```python
from build123d import *

# Parameters (mm, degrees)
SKETCH1_W           = 10
SKETCH1_H           = 7
BOSS_EXTRUDE1_DEPTH = 2
SKETCH2_W           = 7
SKETCH2_H           = 10
BOSS_EXTRUDE2_DEPTH = 2
SKETCH3_R           = 1.05
CUT_EXTRUDE1_DEPTH  = 14.275918047
SKETCH4_R           = 1.05
CUT_EXTRUDE2_DEPTH  = 14.275918047
FILLET1_R           = 1


with BuildPart() as part:
    # Sketch1 → Boss-Extrude1 (new body)
    with BuildSketch(Plane(origin=(0, 0, 0), x_dir=(1, 0, 0), z_dir=(0, 1, 0))):
        with Locations((-5, 0)):
            Rectangle(SKETCH1_W, SKETCH1_H)
    extrude(amount=BOSS_EXTRUDE1_DEPTH)

    # Sketch2 → Boss-Extrude2 (add)
    with BuildSketch(Plane(origin=(0, 0, 0), x_dir=(0, 0, -1), z_dir=(1, 0, 0))):
        with Locations((0, 5)):
            Rectangle(SKETCH2_W, SKETCH2_H)
    extrude(amount=-BOSS_EXTRUDE2_DEPTH)

    # Sketch3 → Cut-Extrude1 (cut, through all)
    with BuildSketch(Plane(origin=(0, 2, 0), x_dir=(1, 0, 0), z_dir=(0, 1, 0))):
        with Locations(Location((-5, 0, 0), (0, 0, 270))):
            Circle(SKETCH3_R)
    extrude(amount=-CUT_EXTRUDE1_DEPTH, mode=Mode.SUBTRACT)

    # Sketch4 → Cut-Extrude2 (cut, through all)
    with BuildSketch(Plane.ZY.offset(2)):
        with Locations((0, 5)):
            Circle(SKETCH4_R)
    extrude(amount=-CUT_EXTRUDE2_DEPTH, mode=Mode.SUBTRACT)

    # Fillet1
    fillet1_edges = [part.edges().sort_by_distance(p)[0] for p in [
        (-10, 2, 0),
        (-6, 2, -3.5),
        (-2, 6, 3.5),
        (-6, 2, 3.5),
        (-2, 6, -3.5),
        (-1, 10, -3.5),
        (-2, 10, 0),
        (-1, 10, 3.5),
        (-2, 2, 0),
        (-10, 1, 3.5),
        (-10, 1, -3.5),
    ]]
    fillet(fillet1_edges, radius=FILLET1_R)


solid = part.part
```
Model file for the job. Use its own axes, mm. A direction names the side the tool comes from. Give positions to 0.01 mm unless a question says otherwise; leave off trailing zeros. Loops run counter-clockwise (first coordinate to the right, second up) from the corner with the lowest first, then second, coordinate; pieces in that order, holes last. Notation, with made-up numbers: (-27, 3.25) - (-19, 3.25) arc R8 cw to (-19, 15.25) - close; hole circle Ø9 at (23, 58). An arc over 180 degrees is marked (long way). One line per item, written item: value. Start each with the question number.
1. Which spindle directions (+Z, -Z, +X, -X, +Y, -Y) get a long thin tool onto all of the face, cutting with end or side? Do faces 1 (the flat face through (-2, 7, 0)), 2 (the cylindrical face through (-9.715, 0.507, -3.199)), 3 (the cylindrical face through (-1.715, 6.042, -3.199)). Say none if no direction does.
2. Pin check, flat tips, straight feed: pin 1 (2.5 mm diameter, centred on y = 5, z = 0, fed in from -X); pin 2 (5 mm diameter, centred on x = -2, y = 6.5, fed in from -Z); pin 3 (1.5 mm diameter, centred on x = -6, z = 0, fed in from +Y); pin 4 (4 mm diameter, centred on x = -4.5, y = 7.5, fed in from +Z). Stop position of each tip, or through.
3. Slice it at B-B (x = -5). List the corners of the cut face in (y, z), plus the area to 3 significant figures.
4. Slice it at D-D (x = -8). List the corners of the cut face in (y, z), plus the area to 3 significant figures.
5. Slice it at A-A (z = 0). List the corners of the cut face in (x, y), plus the area to 3 significant figures.
6. Probe L1, parallel to Y at x = -1.05, z = 0; L2, parallel to X at y = 7, z = 1; L3, parallel to Y at x = -3.5, z = 2.25. List the from-to ranges inside material, lowest first. Write a range as from..to.
7. Slice it at C-C (y = 5). List the corners of the cut face in (x, z), plus the area to 3 significant figures.
8. Pull direction Z, two halves, no side cores. Call faces 4 (the cylindrical face through (-5.958, 1.699, 3.215)), 5 (the cylindrical face through (-5.958, 1.715, -3.199)), 6 (the cylindrical face through (-1.01, 6.04, -0.14)): pulls with the +Z half, pulls with the -Z half, needs draft (parallel to the pull), parting line crosses it, or undercut.
Solution:
1. face 1: +Z, -Z, -X, +Y
1. face 2: -Z, -X, +Y, -Y
1. face 3: -Z, -X, +Y
2. pin 1: stops at x = -2
2. pin 2: stops at z = -3.5
2. pin 3: stops at y = 2
2. pin 4: passes through
3. outline: (0, -3.5) - (1, -3.5) arc R1 ccw to (2, -2.5) - (2, -1.05) - (0, -1.05) - close; (0, 1.05) - (2, 1.05) - (2, 2.5) arc R1 ccw to (1, 3.5) - (0, 3.5) - close
3. area: 9.37 mm^2
4. outline: (0, -3.5) - (1, -3.5) arc R1 ccw to (2, -2.5) - (2, 2.5) arc R1 ccw to (1, 3.5) - (0, 3.5) - close
4. area: 13.6 mm^2
5. outline: (-10, 0) - (-6.05, 0) - (-6.05, 2) - (-9, 2) arc R1 ccw to (-10, 1) - close; (-3.95, 0) - (0, 0) - (0, 3.95) - (-2, 3.95) - (-2, 3) arc R1 cw to (-3, 2) - (-3.95, 2) - close; (-2, 6.05) - (0, 6.05) - (0, 10) - (-1, 10) arc R1 ccw to (-2, 9) - close
5. area: 27.4 mm^2
6. L1: y = 0..3.95, 6.05..10
6. L2: x = -2..0
6. L3: y = 0..2
7. outline: (-2, -2.5) arc R1 ccw to (-1, -3.5) - (0, -3.5) - (0, -1.05) - (-2, -1.05) - close; (-2, 1.05) - (0, 1.05) - (0, 3.5) - (-1, 3.5) arc R1 ccw to (-2, 2.5) - close
7. area: 9.37 mm^2
8. face 4: pulls with the +Z half
8. face 5: pulls with the -Z half
8. face 6: undercut
